```python
from build123d import *

# Parameters (mm, degrees)
F0_W     = 25.4
F0_H     = 17.5
F2_R     = 1.85
F2_R_2   = 4
F3_DEPTH = 40
F4_DEPTH = 5


# Not quite as in the source:
# - a feature names something its author has since deleted; it is built from what else it names


with BuildPart() as f1:
    # F0 (on Right) → F1 (revolve)
    with BuildSketch(Plane.YZ):
        with Locations((12.7, 8.75)):
            Rectangle(F0_W, F0_H)
        Polygon((25.4, 17.5), (25.4, 0), (30.4, 0), (30.4, 40), (25.4, 40), align=None)
    revolve(axis=Axis((0, 12.7, 0), (0, 1, 0)))

    # F2 (on face) → F3 (cut)
    with BuildSketch(Plane(origin=(0, 30.4, 0), x_dir=(-1, 0, 0), z_dir=(0, 1, 0))):
        with Locations((0, 8)):
            Circle(F2_R)
        with Locations((-8, 0)):
            Circle(F2_R)
        Circle(F2_R_2)
        with Locations((0, -8)):
            Circle(F2_R)
        with Locations((8, 0)):
            Circle(F2_R)
    extrude(amount=-F3_DEPTH, mode=Mode.SUBTRACT)

    # F4 (add): a face of the model
    f4_faces = [f1.faces().sort_by_distance(p)[0] for p in [
        (0, 0, -17.0050252532),
    ]]
    extrude(f4_faces, amount=F4_DEPTH)


solid = f1.part
```
Verification items for the finished model (mm, model axes). A direction names the side the tool comes from. Give positions to 0.01 mm unless a question says otherwise; leave off trailing zeros. Loops run counter-clockwise (first coordinate to the right, second up) from the corner with the lowest first, then second, coordinate; pieces in that order, holes last.
1. Go/stop test with flat-tipped pins: pin 1 Ø12 at (y, z) = (25, 20.5) entering from +X; pin 2 Ø10 at (y, z) = (15.5, 16.5) entering from +X; pin 3 Ø2 at (x, z) = (-18.5, -21) entering from -Y; pin 4 Ø3.5 at (x, z) = (8, 0) entering from +Y. Record where each tip stops, or that it passes through.
2. Section check B-B, the plane z = 0. Enter the section's corners in (x, y).
3. Section check C-C, the plane y = 7. Enter the section's corners in (x, z).
4. Section check D-D, the plane z = 8. Enter the section's corners in (x, y).
5. Set-up check for faces 4 (the cylindrical face through (-39.05, 27.86, -8.67)), 5 (the flat face through (-8, 25.4, 17)): record each of +Z, -Z, +X, -X, +Y, -Y from which the full face is reachable in a straight line by a thin tool's end or side.
6. Thickness scan on line 1 (Z direction, x = -8, y = 8); line 2 (Y direction, x = 13, z = -32.5); line 3 (Z direction, x = -7, y = 2). Record the ranges inside material, lowest first.
7. Mould release check, pull along Z, two halves, no side actions. Record for faces 1 (the cylindrical face through (-10.648, 10.413, -13.887)), 2 (the flat face through (-8, 30.4, -8)), 3 (the cylindrical face through (9.468, 12.948, -1.126)): released by +Z, released by -Z, zero draft, split by the parting line, or undercut.
8. Section check A-A, the plane x = 0. Enter the section's corners in (y, z), then the cut area to 3 significant figures.
Geometry says:
1. pin 1: stops at x = 37.27
1. pin 2: stops at x = 13.19
1. pin 3: stops at y = 25.4
1. pin 4: passes through
2. outline: (-40, 25.4) - (-17.5, 25.4) - (-17.5, -5) - (-9.85, -5) - (-9.85, 30.4) - (-40, 30.4) - close; (-6.15, -5) - (-4, -5) - (-4, 30.4) - (-6.15, 30.4) - close; (4, -5) - (6.15, -5) - (6.15, 30.4) - (4, 30.4) - close; (9.85, -5) - (17.5, -5) - (17.5, 25.4) - (40, 25.4) - (40, 30.4) - (9.85, 30.4) - close
3. outline: circle Ø35 at (0, 0); hole circle Ø3.7 at (-8, 0); hole circle Ø8 at (0, 0); hole circle Ø3.7 at (0, -8); hole circle Ø3.7 at (0, 8); hole circle Ø3.7 at (8, 0)
4. outline: (-39.19, 25.4) - (-15.56, 25.4) - (-15.56, -5) - (-1.85, -5) - (-1.85, 30.4) - (-39.19, 30.4) - close; (1.85, -5) - (15.56, -5) - (15.56, 25.4) - (39.19, 25.4) - (39.19, 30.4) - (1.85, 30.4) - close
5. face 4: +Y, -Y
5. face 5: -Y
6. line 1: z = -15.56 to -1.85, 1.85 to 15.56
6. line 2: y = 25.4 to 30.4
6. line 3: z = -16.04 to -1.56, 1.56 to 16.04
7. face 1: split by the parting line
7. face 2: zero draft
7. face 3: undercut
8. outline: (-5, -17.5) - (25.4, -17.5) - (25.4, -40) - (30.4, -40) - (30.4, -9.85) - (-5, -9.85) - close; (-5, -6.15) - (30.4, -6.15) - (30.4, -4) - (-5, -4) - close; (-5, 4) - (30.4, 4) - (30.4, 6.15) - (-5, 6.15) - close; (-5, 9.85) - (30.4, 9.85) - (30.4, 40) - (25.4, 40) - (25.4, 17.5) - (-5, 17.5) - close
8. area: 919 mm2
